Can you work these out from the model? Positions are in its coordinate system, mm. A direction names the side the tool comes from. Round coordinates to 2 decimals unless told otherwise and drop trailing zeros. Order: outer loops, then holes, each group sorted by start corner. A loop starts at its lowest first (then second) coordinate and runs counter-clockwise, first axis right, second up.
Q1. We'd pull the mould along X, two halves only. Please class faces 1 (the face through (38, 357, -4.5)), 2 (the face through (-43.5, 357, 0)), 3 (the face through (-30, 252, 0)): pulls with the +X half, pulls with the -X half, needs draft (parallel to the pull), parting line crosses it, or undercut.
Q2. Will these pins go through, and if not, where does the flat tip stop? P1, Ø25, axis at y = 306.5, z = -19.5, coming from the -X side; P2, Ø8, axis at x = -39, y = 306, coming from the +Z side; P3, Ø8, axis at x = 40.5, y = 395, coming from the -Z side.
Q3. If we section it at A-A (y = 221): Please give me the cut outline in (x, z).
Q4. For faces 4 (the face through (-33.5, 357, 16)), 5 (the face through (33.5, 357, 16)), 6 (the face through (33.5, 357, -16)), 7 (the face through (-39, 357, -4.5)), which set-ups out of +Z, -Z, +X, -X, +Y, -Y let a thin tool reach every point of the face, with its end or its side?
Q5. If I drill on line 1 (X direction, y = 226, z = 22); line 2 (X direction, y = 193.5, z = 2); line 3 (X direction, y = 458, z = 8), over which ranges is the centre line in solid material (lowest first)?
Q6. If we section it at B-B (y = 406.5): Please give me the cut outline in (x, z).
Autodesk Inventor part; units mm, degrees
ref_plane "YZ Plane" through (0, 0, 0) normal (1, 0, 0) x (0, 1, 0)
ref_plane "XZ Plane" through (0, 0, 0) normal (0, 1, 0) x (-1, 0, 0)
ref_plane "XY Plane" through (0, 0, 0) normal (0, 0, 1) x (1, 0, 0)
sketch "草圖1" plane through (0, 0, 0) normal (0, 1, 0) x (-1, 0, 0)
  line L0 (-33.5, 27) -> (33.5, 27)
  line L1 (33.5, 27) -> (33.5, -27)
  line L2 (33.5, -27) -> (-33.5, -27)
  line L3 (-33.5, -27) -> (-33.5, 27)
  line L4 (-33.5, 27) -> (33.5, -27) construction
  line L5 (33.5, 27) -> (-33.5, -27) construction
  line L6 (43.5, -4.5) -> (33.5, -4.5)
  line L7 (33.5, -4.5) -> (33.5, 4.5)
  line L8 (33.5, 4.5) -> (43.5, 4.5)
  line L9 (43.5, 4.5) -> (43.5, -4.5)
  line L10 (-33.5, -4.5) -> (-43.5, -4.5)
  line L11 (-43.5, -4.5) -> (-43.5, 4.5)
  line L12 (-43.5, 4.5) -> (-33.5, 4.5)
  line L13 (-33.5, 4.5) -> (-33.5, -4.5)
  point P0 (0, 0)
  point P1 (33.5, 0)
  point P2 (-33.5, 0)
  point P3 (-33.5, 4.5)
  point P4 (-33.5, -4.5)
  dimension "d0" = 67
  dimension "d1" = 54
  dimension "d2" = 9
  dimension "d3" = 10
extrude "擠出1" add sketch "草圖1" along normal blind 550
sketch "草圖2" plane through (-33.5, 0, 27) normal (0, 0, 1) x (1, 0, 0)
  line L0 (0, 0) -> (0, 550)
  line L1 (0, 550) -> (67, 550)
  line L2 (67, 550) -> (67, 0)
  line L3 (67, 0) -> (0, 0)
  circle A0 centre (33.5, 298) radius 30
  line L4 (3.5, 298) -> (63.5, 298)
  line L5 (63.5, 298) -> (63.5, -29.8228)
  line L6 (63.5, -29.8228) -> (3.5, -29.8228)
  line L7 (3.5, -29.8228) -> (3.5, 298)
  point P0 (33.5, 0)
  point P1 (33.5, 0)
  point P2 (63.5, 298)
  point P3 (3.5, 298)
  dimension "d6" = 298
  dimension "d7" = 60
extrude "擠出2" cut sketch "草圖2" against normal through all contours L7 A0 L5 L3 | L3 L5 L6 L7 | L4 A0 | A0 L4
sketch "草圖3" plane through (-33.5, 550, 27) normal (0, 0, 1) x (1, 0, 0)
  line L0 (-83.0897, -380) -> (150.0897, -380)
  line L1 (150.0897, -380) -> (150.0897, -550)
  line L2 (150.0897, -550) -> (-83.0897, -550)
  line L3 (-83.0897, -550) -> (-83.0897, -380)
  point P0 (33.5, -550)
  point P1 (33.5, -550)
  dimension "d10" = 170
extrude "擠出3" cut sketch "草圖3" against normal through all
sketch "草圖4" plane through (33.5, 550, -27) normal (0, 0, -1) x (-1, 0, 0)
  arc A0 (63.5, -252) -> (3.5, -252) centre (33.5, -252) ccw construction
  circle A1 centre (33.5, -216) radius 30
  line L0 (63.5, -380) -> (3.5, -380)
  line L1 (3.5, -380) -> (3.5, -216)
  line L2 (3.5, -216) -> (63.5, -216)
  line L3 (63.5, -216) -> (63.5, -380)
  point P0 (33.5, -550)
  point P1 (63.5, -380)
  dimension "d13" = 36
  dimension "d14" = 60
sketch "草圖5" plane through (-33.5, 550, 27) normal (0, 0, 1) x (1, 0, 0)
  circle A0 centre (33.5, -214) radius 30
  arc A1 (63.5, -252) -> (3.5, -252) centre (33.5, -252) ccw construction
  line L0 (63.5, -380) -> (3.5, -380)
  line L1 (3.5, -380) -> (3.5, -214)
  line L2 (3.5, -214) -> (63.5, -214)
  line L3 (63.5, -214) -> (63.5, -380)
  point P0 (33.5, -550)
  point P1 (63.5, -380)
  dimension "d15" = 38
  dimension "d16" = 60
loft "斷面混成1" cut profiles "草圖4", "草圖5"
properties part number "Slider-10"
Solution:
1. face 1: needs draft
1. face 2: pulls with the -X half
1. face 3: undercut
2. P1: stops at x = -33.5
2. P2: stops at z = 4.5
2. P3: stops at z = -4.5
3. outline: (-43.5, -4.5) - (-33.5, -4.5) - (-33.5, -27) - (-30, -27) - (-30, 27) - (-33.5, 27) - (-33.5, 4.5) - (-43.5, 4.5) - close; (30, -27) - (33.5, -27) - (33.5, -4.5) - (43.5, -4.5) - (43.5, 4.5) - (33.5, 4.5) - (33.5, 27) - (30, 27) - close
4. face 4: +Z, -X, +Y, -Y
4. face 5: +Z, +X, +Y, -Y
4. face 6: -Z, +X, +Y, -Y
4. face 7: -Z, -X, +Y, -Y
5. line 1: x = -33.5 to -30, 30 to 33.5
5. line 2: x = -43.5 to -30, 30 to 43.5
5. line 3: x = -33.5 to 33.5
6. outline: (-43.5, -4.5) - (-33.5, -4.5) - (-33.5, -27) - (33.5, -27) - (33.5, -4.5) - (43.5, -4.5) - (43.5, 4.5) - (33.5, 4.5) - (33.5, 27) - (-33.5, 27) - (-33.5, 4.5) - (-43.5, 4.5) - close
